The listing builds one solid part. Answer for the finished solid, in the listing's coordinates (mm). Face numbers are marked on the shaded views. Give positions to 0.01 mm unless a question says otherwise; leave off trailing zeros. Write each loop counter-clockwise with the first axis right and the second up, starting at its lowest first coordinate (ties: lowest second). Pieces come first, ordered by that corner, then holes. Notation, with made-up numbers: M 73.5,-7.5 L 115.5,-7.5 A12 ccw 115.5,2.5 Z; hole C 88.5,-20 d9. An arc over 180 degrees is marked long. Answer as a JSON object with one key per item and string values.
Autodesk Inventor part; units mm, degrees
ref_plane "YZ Plane" through (0, 0, 0) normal (1, 0, 0) x (0, 1, 0)
ref_plane "XZ Plane" through (0, 0, 0) normal (0, 1, 0) x (-1, 0, 0)
ref_plane "XY Plane" through (0, 0, 0) normal (0, 0, 1) x (1, 0, 0)
sketch "Sketch1" plane through (0, 0, 0) normal (0, 1, 0) x (-1, 0, 0)
  circle A0 centre (0, 0) radius 15
  dimension "d0" = 30
extrude "Extrusion1" add sketch "Sketch1" along normal blind 26
sketch "Sketch2" plane through (0, 26, 0) normal (0, 1, 0) x (1, 0, 0)
  circle A0 centre (0, 0) radius 2.75
  dimension "d3" = 5.5
extrude "Extrusion2" cut sketch "Sketch2" against normal through all
sketch "Sketch3" plane through (0, 26, 0) normal (0, 1, 0) x (1, 0, 0)
  circle A0 centre (0, 0) radius 20
  dimension "d6" = 40
extrude "Extrusion3" add sketch "Sketch3" along normal blind 0.1
fillet "Fillet1" radius 5 1 edges at (15, 26, 0)
sketch "Sketch4" plane through (0, 0, 0) normal (0, -1, 0) x (1, 0, 0)
  circle A0 centre (0, 0) radius 20
  dimension "d10" = 40
extrude "Extrusion4" add sketch "Sketch4" along normal blind 0.1
fillet "Fillet2" radius 5 1 edges at (15, 0, 0)
properties part number "eje union engrane reductor"
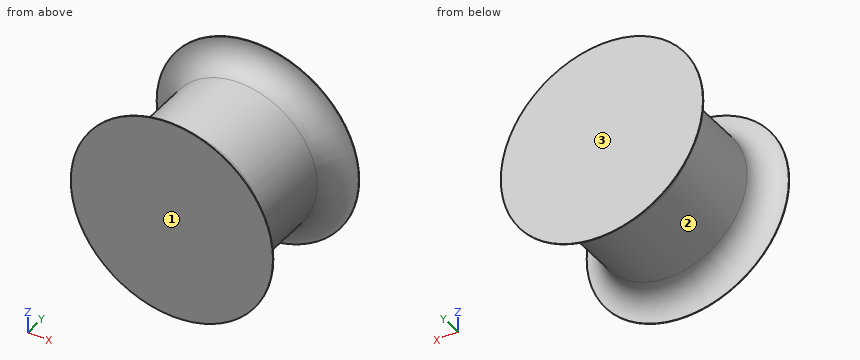
1. A cutting plane is placed at C-C, the plane y = 8. Give the vertices of the cut face in (x, z), plus the area to 3 significant figures.
Verdict:
{"outline": "C 0,0 d30; hole C 0,0 d5.5", "area": "683 mm2"}
2. The mould has two halves that part along Y. Classify the marked faces 1, 2 and 3: released by +Y, released by -Y, zero draft, split by the parting line, or undercut.
Verdict:
{"face 1": "released by -Y", "face 2": "undercut", "face 3": "released by +Y"}
3. A cutting plane is placed at D-D, the plane y = 3. Give the vertices of the cut face in (x, z).
Verdict:
{"outline": "C 0,0 d30.83; hole C 0,0 d5.5"}
4. Flat-ended cylindrical pins translate along their axes: pin 1 (10 mm diameter, centred on y = 8, z = -3, fed in from +X); pin 2 (1.5 mm diameter, centred on y = 13.5, z = 5.5, fed in from +X); pin 3 (1 mm diameter, centred on y = 23, z = -7, fed in from -X). Find the tip coordinate at first contact, or state that the pin passes through.
Verdict:
{"pin 1": "stops at x = 15.25", "pin 2": "stops at x = 14.23", "pin 3": "stops at x = -14.1"}
5. Consider line 1 along Z through (x, y) = (0, 13.75); line 2 along X through (y, z) = (19.5, -1); line 3 along Y through (x, z) = (-4, 18). Determine where each line is inside the solid, lowest interval first.
Verdict:
{"line 1": "z = -15 to -2.75, 2.75 to 15", "line 2": "x = -14.97 to -2.56, 2.56 to 14.97", "line 3": "y = -0.1 to 0.25, 25.75 to 26.1"}
